CAD build for the part. Positions are in the model's coordinates, mm. A direction names the side the tool comes from. Give positions to 0.01 mm unless a question says otherwise; leave off trailing zeros. Order: outer loops, then holes, each group sorted by start corner. A loop starts at its lowest first (then second) coordinate and runs counter-clockwise, first axis right, second up.
```python
from build123d import *

# Parameters (mm, degrees)
SKETCH1_W           = 2000
SKETCH1_H           = 504.823151126
SKETCH1_W_2         = 1151.125401929
SKETCH1_H_2         = 495.176848874
BOSS_EXTRUDE1_DEPTH = 500


with BuildPart() as part:
    # Sketch1 → Boss-Extrude1 (new, symmetric)
    with BuildSketch(Plane(origin=(0, 0, 0), x_dir=(0, 0, -1), z_dir=(1, 0, 0))):
        Rectangle(SKETCH1_W, SKETCH1_H)
        with Locations((424.437299036, 500)):
            Rectangle(SKETCH1_W_2, SKETCH1_H_2)
    extrude(amount=BOSS_EXTRUDE1_DEPTH, both=True)


solid = part.part
```
Item 1: Wall check: L1, parallel to Y at x = 345, z = 489; L2, parallel to Z at x = -207, y = 522.5. Give the ranges that are in metal, low to high.
Item 2: Drop flat-ended pins along their axis: pin 1 Ø1.5 at (x, z) = (-335, 785) entering from +Y; pin 2 Ø6 at (x, y) = (-42, 511) entering from +Z. Give the stop position or say it passes through.
Item 3: Slice it at B-B (z = 670). Give the cut face in (x, y).
Item 4: Tool access for faces 1 (the face through (7, -4, 1000)), 2 (the face through (7, 497, 151.125)): list every direction of +Z, -Z, +X, -X, +Y, -Y with a clear straight run to the whole face (end or side of a thin tool).
Item 5: Slice it at A-A (x = 74.5). Give the cut face in (y, z), and give its area (3 significant figures).
Item 6: Slice it at C-C (y = 631.5). Give the cut face in (x, z).
A:
1. L1: y = -252.41 to 252.41
1. L2: z = -1000 to 151.13
2. pin 1: stops at y = 252.41
2. pin 2: stops at z = 151.13
3. outline: (-500, -252.41) - (500, -252.41) - (500, 252.41) - (-500, 252.41) - close
4. face 1: +Z, +X, -X, +Y, -Y
4. face 2: +Z, +X, -X, +Y
5. outline: (-252.41, -1000) - (747.59, -1000) - (747.59, 151.13) - (252.41, 151.13) - (252.41, 1000) - (-252.41, 1000) - close
5. area: 1,580,000 mm2
6. outline: (-500, -1000) - (500, -1000) - (500, 151.13) - (-500, 151.13) - close
